For this review, take the finished solid that the model builds, in its own axes (mm). A direction names the side the tool comes from. Round coordinates to 2 decimals unless told otherwise and drop trailing zeros. Write each loop counter-clockwise with the first axis right and the second up, starting at its lowest first coordinate (ties: lowest second). Pieces come first, ordered by that corner, then holes. Notation, with made-up numbers: (-39, 54.5) -> (18, 54.5) arc R6 ccw to (18, 63.5) -> close; hole circle Ø1 at (54, 44.5). An arc over 180 degrees is marked (long way). Answer in a Markdown table with one row per item.
from build123d import *

# Parameters (mm, degrees)
SKETCH1_W                    = 20
SKETCH1_H                    = 37
BASE_FLANGE1_DEPTH           = 1
EDGE_FLANGE1_STRIP_W         = 5.4732
EDGE_FLANGE1_STRIP_H         = 1
EDGE_FLANGE1_STRIP_CUT_DEPTH = 20
EDGE_FLANGE1_DEPTH           = 20
SKETCH9_R                    = 2
SKETCH9_R_2                  = 0.9
CUT_EXTRUDE1_DEPTH           = 10
SKETCH10_R                   = 2.25
CUT_EXTRUDE2_DEPTH           = 46.221676218


# Sheet-metal steps are written as plain solids
with BuildPart() as part:
    # Sketch1 → Base-Flange1 (new body)
    with BuildSketch(Plane.XY):
        Rectangle(SKETCH1_W, SKETCH1_H)
    extrude(amount=-BASE_FLANGE1_DEPTH)

    # Edge-Flange1 strip (across the edge) → Edge-Flange1 strip cut (cut)
    with BuildSketch(Plane(origin=(10, 18.5, 0), x_dir=(0, -1, 0), z_dir=(-1, 0, 0))):
        with Locations((-1, -0.5)):
            Rectangle(EDGE_FLANGE1_STRIP_W, EDGE_FLANGE1_STRIP_H)
    edge_flange1_strip_cut = extrude(amount=EDGE_FLANGE1_STRIP_CUT_DEPTH, mode=Mode.SUBTRACT)

    # Edge-Flange1 section (across the edge) → Edge-Flange1 (add)
    with BuildSketch(Plane(origin=(10, 18.5, 0), x_dir=(0, -1, 0), z_dir=(-1, 0, 0))):
        with BuildLine():
            Line((0, 0.7366), (0, 24))
            Line((0, 24), (1, 24))
            Line((1, 24), (1, 0.7366))
            ThreePointArc((1, 0.7366), (1.215745145, 0.215745145), (1.7366, 0))
            Line((1.7366, 0), (1.7366, -1))
            ThreePointArc((1.7366, -1), (0.508638364, -0.491361636), (0, 0.7366))
        make_face()
    edge_flange1 = extrude(amount=EDGE_FLANGE1_DEPTH)

    # Mirror1: Edge-Flange1 strip cut, Edge-Flange1 across plane
    add(edge_flange1_strip_cut.mirror(Plane.ZX), mode=Mode.SUBTRACT)
    add(edge_flange1.mirror(Plane.ZX))

    # Sketch9 → Cut-Extrude1 (cut)
    with BuildSketch(Plane(origin=(0, 0, -1), x_dir=(-1, 0, 0), z_dir=(0, 0, -1))):
        Circle(SKETCH9_R)
        with Locations((-4.5, 0)):
            Circle(SKETCH9_R_2)
        with Locations((4.5, 0)):
            Circle(SKETCH9_R_2)
    extrude(amount=-CUT_EXTRUDE1_DEPTH, mode=Mode.SUBTRACT)

    # Sketch10 → Cut-Extrude2 (cut, through all)
    with BuildSketch(Plane(origin=(0, 18.5, 0), x_dir=(1, 0, 0), z_dir=(0, 1, 0))):
        with Locations(Location((0, -7.5, 0), (0, 0, 270))):
            Circle(SKETCH10_R)
        with Locations(Location((0, -18.5, 0), (0, 0, 270))):
            Circle(SKETCH10_R)
    extrude(amount=-CUT_EXTRUDE2_DEPTH, mode=Mode.SUBTRACT)


solid = part.part
1) Clearance check with a flat-ended pin moving along its axis: pin 1 Ø10 at (x, y) = (1, 1) entering from +Z. State where the tip first meets the part, or that it passes through.
Solved:
| item | result |
|---|---|
| pin 1 | z = 0 |
2) Consider section D-D on x = 0. State how many separate pieces and enclosed holes the cut face has, then the cut area to 3 significant figures.
Solved:
| item | result |
|---|---|
| separate pieces | 6 |
| enclosed holes | 0 |
| area | 61.9 mm² |
3) Consider section C-C on y = 0. State the section outline as (x, z) points, then the cut area to 3 significant figures.
Solved:
| item | result |
|---|---|
| outline | (-10, -1) -> (-5.4, -1) -> (-5.4, 0) -> (-10, 0) -> close; (-3.6, -1) -> (-2, -1) -> (-2, 0) -> (-3.6, 0) -> close; (2, -1) -> (3.6, -1) -> (3.6, 0) -> (2, 0) -> close; (5.4, -1) -> (10, -1) -> (10, 0) -> (5.4, 0) -> close |
| area | 12.4 mm² |
4) Consider section B-B on z = 7.5. State the section outline as (x, y) points.
Solved:
| item | result |
|---|---|
| outline | (-10, -18.5) -> (-2.25, -18.5) -> (-2.25, -17.5) -> (-10, -17.5) -> close; (-10, 17.5) -> (-2.25, 17.5) -> (-2.25, 18.5) -> (-10, 18.5) -> close; (2.25, -18.5) -> (10, -18.5) -> (10, -17.5) -> (2.25, -17.5) -> close; (2.25, 17.5) -> (10, 17.5) -> (10, 18.5) -> (2.25, 18.5) -> close |
5) For line 1 (Y direction, x = 7, z = 5.5); line 2 (X direction, y = 18.1, z = 7.5); line 3 (Z direction, x = 1, y = -13.5), list the stretches that pass through material, from the lowest coordinate up. Write a range as [from, to].
Solved:
| item | result |
|---|---|
| line 1 | [-18.5, -17.5], [17.5, 18.5] |
| line 2 | [-10, -2.25], [2.25, 10] |
| line 3 | [-1, 0] |
6) Consider section A-A on x = 4.5. State the section outline as (y, z) points.
Solved:
| item | result |
|---|---|
| outline | (-18.5, 0.74) arc R1.74 ccw to (-16.76, -1) -> (-0.9, -1) -> (-0.9, 0) -> (-16.76, 0) arc R0.74 cw to (-17.5, 0.74) -> (-17.5, 24) -> (-18.5, 24) -> close; (0.9, -1) -> (16.76, -1) arc R1.74 ccw to (18.5, 0.74) -> (18.5, 24) -> (17.5, 24) -> (17.5, 0.74) arc R0.74 cw to (16.76, 0) -> (0.9, 0) -> close |
7) For faces 4 (the flat face through (0, 18.5, 12)), 5 (the flat face through (-2.4, 0.2, 0)), list the 3-axis set-ups (+Z, -Z, +X, -X, +Y, -Y) from which the entire face can be reached by the end or side of a thin tool; tool diameter is ignored.
Solved:
| item | result |
|---|---|
| face 4 | +Z, -Z, +X, -X, +Y |
| face 5 | +Z, +X, -X |
8) Mouldability with a two-part tool opening along Z and no side actions: class faces 1 (the flat face through (0, -18, 24)), 2 (the cylindrical face through (0.676, 18.007, 20.646)), 3 (the cylindrical face through (-3.6, 0, -0.5)) as pulls with the +Z half, pulls with the -Z half, needs draft (parallel to the pull), parting line crosses it, or undercut.
Solved:
| item | result |
|---|---|
| face 1 | pulls with the +Z half |
| face 2 | undercut |
| face 3 | needs draft |
